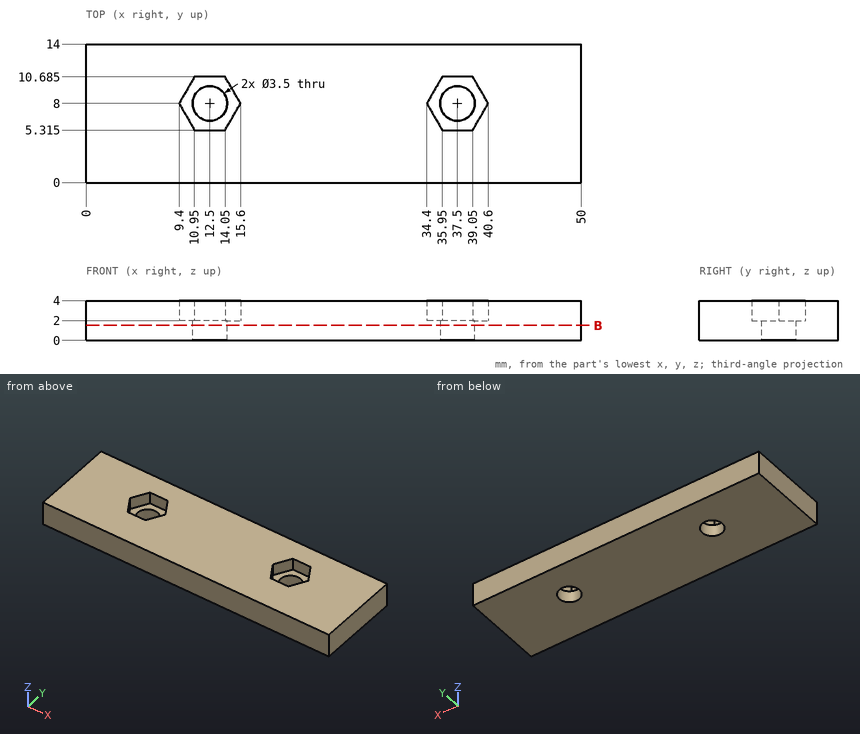
For this review, use the dimensioned drawing (mm, ordinates from the lowest corner) and the shaded views. Coordinates: 2 decimals unless noted, no trailing zeros. Loops run counter-clockwise (first coordinate to the right, second up) from the corner with the lowest first, then second, coordinate; pieces in that order, holes last. Notation, with made-up numbers: M -0.75,77.5 L 51.25,77.5 A13 ccw 51.25,95.5 Z; hole C 0.25,59 d11. An arc over 180 degrees is marked long. Answer as CSV lines item,"result".
Item 1: Add section B-B on z = 1.5. State the section outline as (x, y) points.
Answer list:
outline,"M 0,0 L 50,0 L 50,14 L 0,14 Z; hole C 12.5,8 d3.5; hole C 37.5,8 d3.5"
Item 2: For probe 1 along X at (y, z) = (8, 0.75); probe 2 along Y at (x, z) = (37.5, 0.85); probe 3 along X at (y, z) = (7, 3.1), list the stretches that pass through material, from the lowest coordinate up.
Answer list:
probe 1,"0 to 10.75, 14.25 to 35.75, 39.25 to 50"
probe 2,"0 to 6.25, 9.75 to 14"
probe 3,"0 to 9.98, 15.02 to 34.98, 40.02 to 50"
Item 3: For P1, Ø1.6, axis at x = 38.5, y = 7, coming from the +Z side; P2, Ø3, axis at x = 12.5, y = 8, coming from the -Z side, all flat-tipped, find the tip position at first contact; note any pin that passes through.
Answer list:
P1,"z = 2"
P2,"through"
